Design review of the part built by this model. Coordinates are the model's own, in mm. Coordinates: 2 decimals unless noted, no trailing zeros. Write each loop counter-clockwise with the first axis right and the second up, starting at its lowest first coordinate (ties: lowest second). Pieces come first, ordered by that corner, then holes.
Q1. Take a section at A-A, the plane z = 1.15. Write out the cut boundary in (x, y).
Q2. Take a section at C-C, the plane y = 59. Write out the cut boundary in (x, z), plus the area to 3 significant figures.
Q3. Take a section at B-B, the plane x = -33.5. Write out the cut boundary in (y, z).
Q4. Take a section at D-D, the plane x = -11. Write out the cut boundary in (y, z), plus the area to 3 significant figures.
Q5. For L1, parallel to X at y = 43, z = 3.7; L2, parallel to Y at x = -26, z = 4.45; L3, parallel to Y at x = -35, z = 4.65, list the stretches that pass through material, from the lowest coordinate up.
Q6. For pin 1 Ø3.5 at (x, y) = (-33.88, 53.9) entering from -Z; pin 2 Ø2.5 at (y, z) = (43, 2.5) entering from +X; pin 3 Ø5 at (x, y) = (6.12, 53.9) entering from -Z, all flat-tipped, find the tip position at first contact; note any pin that passes through.
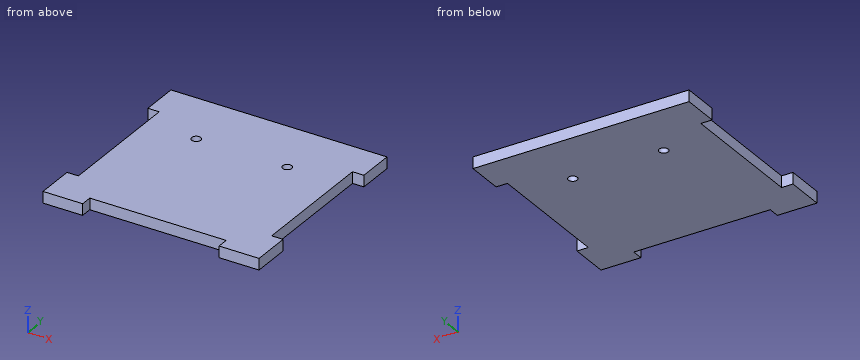
from build123d import *

# Parameters (mm, degrees)
SKIZZE1_R                       = 2
AUFSATZ_LINEAR_AUSTRAGEN1_DEPTH = 5


with BuildPart() as part:
    # Skizze1 → Aufsatz-Linear austragen1 (new body)
    # profile 1 of 4: a face of its own
    with BuildSketch(Plane.XY):
        Polygon((-56.378328771, 75.078341375), (-56.378328771, 63.819239112), (-56.378328771, 6.977133849), (-56.378328771, -4.921658625), (-43.939454059, -4.921658625), (16.060545941, -4.921658625), (28.621671229, -4.921658625), (28.621671229, 6.977133849), (28.621671229, 63.819239112), (28.621671229, 75.078341375), align=None)
        with Locations((-33.878328771, 53.901870786)):
            Circle(SKIZZE1_R, mode=Mode.SUBTRACT)
        with Locations((6.121671229, 53.901870786)):
            Circle(SKIZZE1_R, mode=Mode.SUBTRACT)
    # profile 2 of 4: a face of its own
    with BuildSketch(Plane.XY):
        Polygon((-61.378328771, 80.078341375), (-61.378328771, 63.819239112), (-56.378328771, 63.819239112), (-56.378328771, 75.078341375), (28.621671229, 75.078341375), (28.621671229, 63.819239112), (33.621671229, 63.819239112), (33.621671229, 80.078341375), align=None)
    # profile 3 of 4: a face of its own
    with BuildSketch(Plane.XY):
        Polygon((-56.378328771, -4.921658625), (-56.378328771, 6.977133849), (-61.378328771, 6.977133849), (-61.378328771, -9.921658625), (-43.939454059, -9.921658625), (-43.939454059, -4.921658625), align=None)
    # profile 4 of 4: a face of its own
    with BuildSketch(Plane.XY):
        Polygon((33.621671229, 6.977133849), (28.621671229, 6.977133849), (28.621671229, -4.921658625), (16.060545941, -4.921658625), (16.060545941, -9.921658625), (33.621671229, -9.921658625), align=None)
    extrude(amount=AUFSATZ_LINEAR_AUSTRAGEN1_DEPTH)


solid = part.part
Responses:
1. outline: (-61.38, -9.92) - (-43.94, -9.92) - (-43.94, -4.92) - (16.06, -4.92) - (16.06, -9.92) - (33.62, -9.92) - (33.62, 6.98) - (28.62, 6.98) - (28.62, 63.82) - (33.62, 63.82) - (33.62, 80.08) - (-61.38, 80.08) - (-61.38, 63.82) - (-56.38, 63.82) - (-56.38, 6.98) - (-61.38, 6.98) - close; hole circle Ø4 at (-33.88, 53.9); hole circle Ø4 at (6.12, 53.9)
2. outline: (-56.38, 0) - (28.62, 0) - (28.62, 5) - (-56.38, 5) - close
2. area: 425 mm2
3. outline: (-4.92, 0) - (51.94, 0) - (51.94, 5) - (-4.92, 5) - close; (55.87, 0) - (80.08, 0) - (80.08, 5) - (55.87, 5) - close
4. outline: (-4.92, 0) - (80.08, 0) - (80.08, 5) - (-4.92, 5) - close
4. area: 425 mm2
5. L1: x = -56.38 to 28.62
5. L2: y = -4.92 to 80.08
5. L3: y = -4.92 to 52.25, 55.56 to 80.08
6. pin 1: passes through
6. pin 2: stops at x = 28.62
6. pin 3: stops at z = 0
